Design review of the part shown in the three views and the two pictorial views. Dimensions are in mm from the part's minimum x, y and z. Coordinates: 2 decimals unless noted, no trailing zeros. Loops run counter-clockwise (first coordinate to the right, second up) from the corner with the lowest first, then second, coordinate; pieces in that order, holes last.
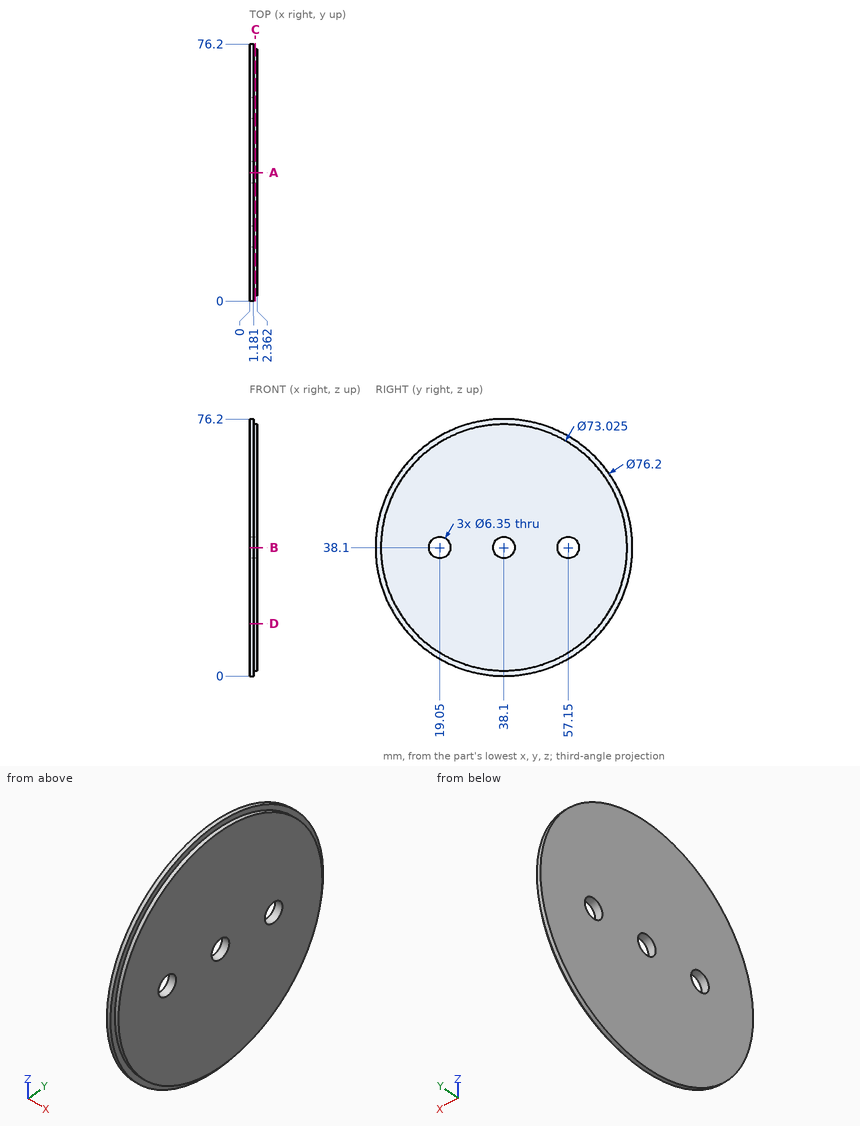
Q1. Wall thickness on probe 1 along Y at (x, z) = (1.25, 38.1) (1 decimal); probe 2 along Y at (x, z) = (0.6, 38.1) (3 decimals); probe 3 along X at (y, z) = (12, 65.5): over which ranges is each line inside the solid? List them lowest first.
Q2. Consider section A-A (y = 38.1). State the section outline as (x, z) points (1 decimal), then the cut area to 3 significant figures.
Q3. Consider section B-B (z = 38.1). State the section outline as (x, y) points (1 decimal), then the cut area to 3 significant figures.
Q4. Consider section C-C (x = 1.7). Count the separate pieces of the cut face and the enclosed holes in it, then the cut area to 3 significant figures.
Q5. For pin 1 Ø4 at (y, z) = (19.05, 38.1) entering from -X, flat-tipped, find the tip position at first contact; note if it passes through.
Q6. Consider section D-D (z = 15.5). State the section outline as (x, y) points.
Model answer:
1. probe 1: y = 1.6 to 15.9, 22.2 to 34.9, 41.3 to 54, 60.3 to 74.6
1. probe 2: y = 0 to 15.875, 22.225 to 34.925, 41.275 to 53.975, 60.325 to 76.2
1. probe 3: x = 0 to 1.18
2. outline: (0, 0) - (1.2, 0) - (1.2, 1.6) - (2.4, 1.6) - (2.4, 34.9) - (0, 34.9) - close; (0, 41.3) - (2.4, 41.3) - (2.4, 74.6) - (1.2, 74.6) - (1.2, 76.2) - (0, 76.2) - close
2. area: 161 mm2
3. outline: (0, 0) - (1.2, 0) - (1.2, 1.6) - (2.4, 1.6) - (2.4, 15.9) - (0, 15.9) - close; (0, 22.2) - (2.4, 22.2) - (2.4, 34.9) - (0, 34.9) - close; (0, 41.3) - (2.4, 41.3) - (2.4, 54) - (0, 54) - close; (0, 60.3) - (2.4, 60.3) - (2.4, 74.6) - (1.2, 74.6) - (1.2, 76.2) - (0, 76.2) - close
3. area: 131 mm2
4. separate pieces: 1
4. enclosed holes: 3
4. area: 4,090 mm2
5. pin 1: passes through
6. outline: (0, 7.43) - (1.18, 7.43) - (1.18, 9.42) - (2.36, 9.42) - (2.36, 66.78) - (1.18, 66.78) - (1.18, 68.77) - (0, 68.77) - close
